Geometry check sheet. Reference: the model listing, model coordinates, mm. A direction names the side the tool comes from. Coordinates: 2 decimals unless noted, no trailing zeros. Write each loop counter-clockwise with the first axis right and the second up, starting at its lowest first coordinate (ties: lowest second). Pieces come first, ordered by that corner, then holes. Notation, with made-up numbers: M 20,2 L 28,2 A19 cw 28,10 Z; hole C -10,2.5 d8. An arc over 180 degrees is marked long. Write item = value, one per line. Start each with the question number.
Autodesk Inventor part; units mm, degrees
ref_plane "Work Plane1" through (0, 0, -20) normal (0, 0, 1) x (1, 0, 0)
ref_plane "YZ Plane" through (0, 0, 0) normal (1, 0, 0) x (0, 1, 0)
ref_plane "XZ Plane" through (0, 0, 0) normal (0, 1, 0) x (-1, 0, 0)
sketch "Sketch1" plane through (0, 0, 0) normal (0, 1, 0) x (-1, 0, 0)
  line L0 (0, 170) -> (0, 0)
  line L1 (-195, -25) -> (-25, -25)
  line L2 (-220, 0) -> (-220, 170)
  line L3 (-25, 195) -> (-195, 195)
  line L4 (-25, 195) -> (0, 195)
  line L5 (0, 195) -> (0, 170)
  line L6 (0, 0) -> (0, -25)
  line L7 (0, -25) -> (-25, -25)
  line L8 (-195, -25) -> (-220, -25)
  line L9 (-220, -25) -> (-220, 0)
  line L10 (-220, 170) -> (-220, 195)
  line L11 (-195, 195) -> (-220, 195)
  line L12 (-25, 170) -> (-195, 170)
  line L13 (-195, 170) -> (-195, 0)
  line L14 (-195, 0) -> (-25, 0)
  line L15 (-25, 0) -> (-25, 170)
  line L16 (-25, 170) -> (-195, 0) construction
  line L17 (-195, 170) -> (-25, 0) construction
  point P0 (-110, 85)
  dimension "d2" = 170
  dimension "d5" = 170
  dimension "d7" = 170
  dimension "d8" = 170
extrude "Extrusion1" add sketch "Sketch1" along normal blind 25
ref_plane "Work Plane1" through (0, 0, -20) normal (0, 0, 1) x (1, 0, 0)
sketch "Sketch2" plane through (0, 0, -20) normal (0, 0, 1) x (1, 0, 0)
  line L0 (0, 0) -> (0, 25)
  circle A0 centre (10, 12.5) radius 1.5
  line L1 (220, 0) -> (220, 25)
  circle A1 centre (210, 12.5) radius 1.5
extrude "Extrusion2" cut sketch "Sketch2" along normal through all both and the other way through all
sketch "Sketch3" plane through (0, 0, 195) normal (0, 0, 1) x (1, 0, 0)
  line L0 (195, 25) -> (25, 25)
  circle A0 centre (110, 12.5) radius 1.5
hole "Hole1" at (110, 12.5, 195) direction (0, 0, -1) diameter 3 end through all
properties part number "sambung kotak"
Q1. Cross-section at B-B on z = 38. Enter the section's corners in (x, y).
Q2. Scan lines: L1, parallel to X at y = 12.75, z = 28; L2, parallel to X at y = 12.5, z = -18.5; L3, parallel to Z at x = 112.5, y = 9.25. Record each from-to range of solid material in increasing order.
Q3. Draft check along Z on faces 1 (the face through (109, 10, 170)), 2 (the face through (25, 12, 84)), 3 (the face through (0, 12, 87)), 4 (the face through (112, 12, 195)). Enter one of: pulls with the +Z half, pulls with the -Z half, needs draft (parallel to the pull), parting line crosses it, or undercut.
Q4. Cross-section at C-C on y = 6.25. Enter the section's corners in (x, z).
Q5. Gauge pin test, flat end, axial feed: pin 1 (1.8 mm diameter, centred on x = 110, y = 12.5, fed in from +Z). Record the tip position at first contact, or that the pin passes through.
Q6. Cross-section at A-A on x = 156.5. Enter the section's corners in (y, z).
Q7. Set-up check for faces 5 (the face through (14, 25, 87)), 6 (the face through (195, 12, 86)): record each of +Z, -Z, +X, -X, +Y, -Y from which the full face is reachable in a straight line by a thin tool's end or side.
Values found:
q1.outline = M 0,0 L 25,0 L 25,25 L 0,25 Z; M 195,0 L 220,0 L 220,25 L 195,25 Z; hole C 10,12.5 d3; hole C 210,12.5 d3
q2.L1 = 0 to 8.52, 11.48 to 25, 195 to 208.52, 211.48 to 220
q2.L2 = 0 to 8.5, 11.5 to 108.5, 111.5 to 208.5, 211.5 to 220
q2.L3 = -25 to 0, 170 to 195
q3.face_1 = undercut
q3.face_2 = undercut
q3.face_3 = needs draft
q3.face_4 = pulls with the +Z half
q4.outline = M 0,-25 L 220,-25 L 220,195 L 0,195 Z; hole M 25,0 L 195,0 L 195,170 L 25,170 Z
q5.pin_1 = through
q6.outline = M 0,-25 L 25,-25 L 25,0 L 0,0 Z; M 0,170 L 25,170 L 25,195 L 0,195 Z
q7.face_5 = +Z, -Z, +X, -X, +Y
q7.face_6 = +Y, -Y
